```python
from build123d import *

# Parameters (mm, degrees)
SKETCH_1_W          = 45
SKETCH_1_H          = 5
EXTRUDE_1_DEPTH     = 4
SKETCH_2_W          = 125
SKETCH_2_H          = 92.025
SKETCH_2_R          = 1.5
SKETCH_2_R_2        = 1.35
SKETCH_2_W_2        = 59.93870536
SKETCH_2_H_2        = 40.423778034
SKETCH_2_W_3        = 45
SKETCH_2_H_3        = 5
EXTRUDE_2_DEPTH     = 4
CUT_EXTRUDE_1_DEPTH = 4
FILLET_1_R          = 5
FILLET_2_R          = 1
CUT_EXTRUDE_START   = -1.5
SKETCH_4_R          = 2.85
SKETCH_4_R_2        = 1.35
SKETCH_4_R_3        = 3
SKETCH_4_R_4        = 1.5
CUT_EXTRUDE_2_DEPTH = 1.5


with BuildPart() as part:
    # 草图1 → 凸台-拉伸1 (new body)
    with BuildSketch(Plane.XY):
        Rectangle(SKETCH_1_W, SKETCH_1_H)
    extrude(amount=EXTRUDE_1_DEPTH)

    # 草图2 → 凸台-拉伸2 (add)
    # profile 1 of 2: a face of its own
    with BuildSketch(Plane(origin=(0, 0, 0), x_dir=(-1, 0, 0), z_dir=(0, 0, -1))):
        with Locations((0, 48.5125)):
            Rectangle(SKETCH_2_W, SKETCH_2_H)
        with Locations((-57.5, 89.525)):
            Circle(SKETCH_2_R, mode=Mode.SUBTRACT)
        with Locations((57.5, 89.525)):
            Circle(SKETCH_2_R, mode=Mode.SUBTRACT)
        with Locations((-43, 80.5)):
            Circle(SKETCH_2_R_2, mode=Mode.SUBTRACT)
        with Locations((43, 80.5)):
            Circle(SKETCH_2_R_2, mode=Mode.SUBTRACT)
        with Locations((43, 22.5)):
            Circle(SKETCH_2_R_2, mode=Mode.SUBTRACT)
        with Locations((-43, 22.5)):
            Circle(SKETCH_2_R_2, mode=Mode.SUBTRACT)
        with BuildLine():
            Line((-52.5, 68.5125), (-52.5, 28.5125))
            ThreePointArc((-52.5, 28.5125), (-55.5, 25.5125), (-58.5, 28.5125))
            Line((-58.5, 28.5125), (-58.5, 68.5125))
            ThreePointArc((-58.5, 68.5125), (-55.5, 71.5125), (-52.5, 68.5125))
        make_face(mode=Mode.SUBTRACT)
        with BuildLine():
            Line((58.5, 68.5125), (58.5, 28.5125))
            ThreePointArc((58.5, 28.5125), (55.5, 25.5125), (52.5, 28.5125))
            Line((52.5, 28.5125), (52.5, 68.5125))
            ThreePointArc((52.5, 68.5125), (55.5, 71.5125), (58.5, 68.5125))
        make_face(mode=Mode.SUBTRACT)
        with Locations((0, 51.5)):
            Rectangle(SKETCH_2_W_2, SKETCH_2_H_2, mode=Mode.SUBTRACT)
        with BuildLine():
            Line((-48.597194221, 12.5), (-23.597194221, 12.5))
            ThreePointArc((-23.597194221, 12.5), (-20.597194221, 9.5), (-23.597194221, 6.5))
            Line((-23.597194221, 6.5), (-48.597194221, 6.5))
            ThreePointArc((-48.597194221, 6.5), (-51.597194221, 9.5), (-48.597194221, 12.5))
        make_face(mode=Mode.SUBTRACT)
        with BuildLine():
            Line((48.597194221, 12.5), (23.597194221, 12.5))
            ThreePointArc((23.597194221, 12.5), (20.597194221, 9.5), (23.597194221, 6.5))
            Line((23.597194221, 6.5), (48.597194221, 6.5))
            ThreePointArc((48.597194221, 6.5), (51.597194221, 9.5), (48.597194221, 12.5))
        make_face(mode=Mode.SUBTRACT)
    # profile 2 of 2: a face of its own
    with BuildSketch(Plane(origin=(0, 0, 0), x_dir=(-1, 0, 0), z_dir=(0, 0, -1))):
        Rectangle(SKETCH_2_W_3, SKETCH_2_H_3)
    extrude(amount=-EXTRUDE_2_DEPTH)

    # 草图3 → 切除-拉伸1 (cut)
    with BuildSketch(Plane(origin=(0, 0, 0), x_dir=(-1, 0, 0), z_dir=(0, 0, -1))):
        with BuildLine():
            Line((-23.5, 2.5), (-22.5, 2.5))
            Line((-22.5, 2.5), (-22.5, 1.5))
            ThreePointArc((-22.5, 1.5), (-21.792893219, 1.792893219), (-21.5, 2.5))
            ThreePointArc((-21.5, 2.5), (-22.5, 3.5), (-23.5, 2.5))
        make_face()
        with BuildLine():
            Line((-22.5, 1.5), (-22.5, 2.5))
            Line((-22.5, 2.5), (-23.5, 2.5))
            ThreePointArc((-23.5, 2.5), (-23.207106781, 1.792893219), (-22.5, 1.5))
        make_face()
        with BuildLine():
            ThreePointArc((23.5, 2.5), (21.792893219, 3.207106781), (22.5, 1.5))
            Line((22.5, 1.5), (22.5, 2.5))
            Line((22.5, 2.5), (23.5, 2.5))
        make_face()
        with BuildLine():
            Line((22.5, 2.5), (22.5, 1.5))
            ThreePointArc((22.5, 1.5), (23.207106781, 1.792893219), (23.5, 2.5))
            Line((23.5, 2.5), (22.5, 2.5))
        make_face()
    extrude(amount=-CUT_EXTRUDE_1_DEPTH, mode=Mode.SUBTRACT)

    # 圆角1
    fillet_1_edges = [part.edges().sort_by_distance(p)[0] for p in [
        (-62.5, 2.5, 2),
        (-29.96935268, 71.711889017, 2),
        (29.96935268, 71.711889017, 2),
        (29.96935268, 31.288110983, 2),
        (62.5, 94.525, 2),
        (-62.5, 94.525, 2),
        (-29.96935268, 31.288110983, 2),
        (62.5, 2.5, 2),
    ]]
    fillet(fillet_1_edges, radius=FILLET_1_R)

    # 圆角2
    fillet_2_edges = [part.edges().sort_by_distance(p)[0] for p in [
        (22.5, -2.5, 2),
        (-22.5, -2.5, 2),
    ]]
    fillet(fillet_2_edges, radius=FILLET_2_R)

    # 草图4 → 切除-拉伸2 (cut)
    # profile 1 of 6: a face of its own
    with BuildSketch(Plane.XY.offset(4).offset(CUT_EXTRUDE_START)):
        with Locations((43, 22.5)):
            Circle(SKETCH_4_R)
        with Locations(Location((43, 22.5, 0), (0, 0, 180))):
            Circle(SKETCH_4_R_2, mode=Mode.SUBTRACT)
    # profile 2 of 6: a face of its own
    with BuildSketch(Plane.XY.offset(4).offset(CUT_EXTRUDE_START)):
        with Locations((43, 80.5)):
            Circle(SKETCH_4_R)
        with Locations(Location((43, 80.5, 0), (0, 0, 180))):
            Circle(SKETCH_4_R_2, mode=Mode.SUBTRACT)
    # profile 3 of 6: a face of its own
    with BuildSketch(Plane.XY.offset(4).offset(CUT_EXTRUDE_START)):
        with Locations((-43, 22.5)):
            Circle(SKETCH_4_R)
        with Locations(Location((-43, 22.5, 0), (0, 0, 180))):
            Circle(SKETCH_4_R_2, mode=Mode.SUBTRACT)
    # profile 4 of 6: a face of its own
    with BuildSketch(Plane.XY.offset(4).offset(CUT_EXTRUDE_START)):
        with Locations((-43, 80.5)):
            Circle(SKETCH_4_R)
        with Locations(Location((-43, 80.5, 0), (0, 0, 180))):
            Circle(SKETCH_4_R_2, mode=Mode.SUBTRACT)
    # profile 5 of 6: a face of its own
    with BuildSketch(Plane.XY.offset(4).offset(CUT_EXTRUDE_START)):
        with Locations((57.5, 89.525)):
            Circle(SKETCH_4_R_3)
        with Locations(Location((57.5, 89.525, 0), (0, 0, 180))):
            Circle(SKETCH_4_R_4, mode=Mode.SUBTRACT)
    # profile 6 of 6: a face of its own
    with BuildSketch(Plane.XY.offset(4).offset(CUT_EXTRUDE_START)):
        with Locations((-57.5, 89.525)):
            Circle(SKETCH_4_R_3)
        with Locations(Location((-57.5, 89.525, 0), (0, 0, 180))):
            Circle(SKETCH_4_R_4, mode=Mode.SUBTRACT)
    extrude(amount=CUT_EXTRUDE_2_DEPTH, mode=Mode.SUBTRACT)


solid = part.part
```
Model file for the job. Use its own axes, mm. A direction names the side the tool comes from. Give positions to 0.01 mm unless a question says otherwise; leave off trailing zeros. Loops run counter-clockwise (first coordinate to the right, second up) from the corner with the lowest first, then second, coordinate; pieces in that order, holes last. Notation, with made-up numbers: (74, 62) -> (94, 62) arc R17 cw to (94, 92) -> close; hole circle Ø8 at (58.25, 65.25). An arc over 180 degrees is marked (long way). Write each question's results on one line, items separated by ' | '.
(1) Cut at C-C on y = 22.5. List the corners of the cut face in (x, z).
Geometry results:
outline: (-62.5, 0) -> (-44.35, 0) -> (-44.35, 2.5) -> (-45.85, 2.5) -> (-45.85, 4) -> (-62.5, 4) -> close; (-41.65, 0) -> (41.65, 0) -> (41.65, 2.5) -> (40.15, 2.5) -> (40.15, 4) -> (-40.15, 4) -> (-40.15, 2.5) -> (-41.65, 2.5) -> close; (44.35, 0) -> (62.5, 0) -> (62.5, 4) -> (45.85, 4) -> (45.85, 2.5) -> (44.35, 2.5) -> close
(2) Cut at D-D on z = 1.7. Give the number of separate pieces and of enclosed holes in the cut face, and give its area (3 significant figures).
Geometry results:
separate pieces: 1 | enclosed holes: 11 | area: 8,370 mm²
(3) Cut at B-B on x = 1.5. List the corners of the cut face in (y, z) (3 decimals).
Geometry results:
outline: (-2.5, 0) -> (31.288, 0) -> (31.288, 4) -> (-2.5, 4) -> close; (71.712, 0) -> (94.525, 0) -> (94.525, 4) -> (71.712, 4) -> close
(4) Tool access for faces 1 (the cylindrical face through (55.434, 25.513, 1.972)), 2 (the flat face through (0, -2.5, 2)), 3 (the cylindrical face through (-59.711, 91.553, 3.24)): list every direction of +Z, -Z, +X, -X, +Y, -Y with a clear straight run to the whole face (end or side of a thin tool).
Geometry results:
face 1: +Z, -Z | face 2: +Z, -Z, +X, -X, -Y | face 3: +Z
(5) Cut at A-A on y = 52. List the corners of the cut face in (x, z), and give its area (3 significant figures).
Geometry results:
outline: (-62.5, 0) -> (-58.5, 0) -> (-58.5, 4) -> (-62.5, 4) -> close; (-52.5, 0) -> (-29.97, 0) -> (-29.97, 4) -> (-52.5, 4) -> close; (29.97, 0) -> (52.5, 0) -> (52.5, 4) -> (29.97, 4) -> close; (58.5, 0) -> (62.5, 0) -> (62.5, 4) -> (58.5, 4) -> close | area: 212 mm²
(6) Probe line 1 along Y through (x, z) = (43, 3.05) (3 decimals); line 2 along Y through (x, z) = (-25, 3.45) (3 decimals); line 3 along Y through (x, z) = (43, 1.7) (3 decimals). List the from-to ranges inside material, lowest first.
Geometry results:
line 1: y = 2.5 to 6.5, 12.5 to 19.65, 25.35 to 77.65, 83.35 to 94.525 | line 2: y = 2.5 to 6.5, 12.5 to 31.288, 71.712 to 94.525 | line 3: y = 2.5 to 6.5, 12.5 to 21.15, 23.85 to 79.15, 81.85 to 94.525
(7) Pull direction Y, two halves, no side cores. Call faces 4 (the flat face through (-22.5, 0, 2)), 5 (the cylindrical face through (-61.07, 4, 2.03)), 6 (the cylindrical face through (-55.566, 25.513, 1.972)): released by +Y, released by -Y, zero draft, split by the parting line, or undercut.
Geometry results:
face 4: zero draft | face 5: released by -Y | face 6: undercut
(8) Flat gauge pins, fed straight in: pin 1 Ø1.2 at (x, z) = (-32, 2.5) entering from -Y; pin 2 Ø4.5 at (x, y) = (43.5, 80.5) entering from +Z; pin 3 Ø0.9 at (y, z) = (-0.5, 2) entering from -X. Where does each tip first touch, or does it go through?
Geometry results:
pin 1: stops at y = 2.5 | pin 2: stops at z = 2.5 | pin 3: stops at x = -22.5
